Autodesk Inventor part; units mm, degrees
ref_plane "YZ Plane" through (0, 0, 0) normal (1, 0, 0) x (0, 1, 0)
ref_plane "XZ Plane" through (0, 0, 0) normal (0, 1, 0) x (-1, 0, 0)
ref_plane "XY Plane" through (0, 0, 0) normal (0, 0, 1) x (1, 0, 0)
sketch "Эскиз1" plane through (0, 0, 0) normal (0, 0, 1) x (1, 0, 0)
  line L0 (0, 0) -> (5.4, 0)
  line L1 (5.4, 0) -> (5.4, 4.4)
  line L2 (5.4, 4.4) -> (0, 4.4)
  line L3 (0, 4.4) -> (0, 0)
  dimension "d0" = 5.4
  dimension "d1" = 4.4
extrude "Выдавливание1" add sketch "Эскиз1" along normal blind 2
sketch "Эскиз2" plane through (0, 0, 2) normal (0, 0, 1) x (1, 0, 0)
  line L0 (0, 0) -> (5.4, 0)
  line L1 (5.4, 0) -> (5.4, 4.4)
  line L2 (5.4, 4.4) -> (0, 4.4)
  line L3 (0, 4.4) -> (0, 0)
  line L4 (0.3, 3.95) -> (5.1, 3.95)
  line L5 (5.1, 3.95) -> (5.1, 0.45)
  line L6 (5.1, 0.45) -> (0.3, 0.45)
  line L7 (0.3, 0.45) -> (0.3, 3.95)
  line L8 (-0.7, 4.95) -> (6.1, 4.95)
  line L9 (6.1, 4.95) -> (6.1, -0.55)
  line L10 (6.1, -0.55) -> (-0.7, -0.55)
  line L11 (-0.7, -0.55) -> (-0.7, 4.95)
  dimension "d4" = 4.8
  dimension "d5" = 3.5
  dimension "d6" = 5.4
  dimension "d7" = 4.4
  dimension "d8" = 0.3
  dimension "d9" = 0.45
  dimension "d12" = 1
  dimension "d13" = 1
  dimension "d14" = 1
  dimension "d15" = 1
extrude "Выдавливание3" add sketch "Эскиз2" along normal blind 1.5 contours L3 L2 L1 L0 | L8 L9 L10 L11
equation "\"d8\" = -0.5 * d4 + 0.5 * d6"
equation "\"d9\" = -0.5 * d5 + 0.5 * d7"
equation "\"d13\" = d12"
equation "\"d14\" = d12"
equation "\"d15\" = d12"
properties part number "button"
The listing builds one solid part. Answer for the finished solid, in the listing's coordinates (mm). A direction names the side the tool comes from. Coordinates: 2 decimals unless noted, no trailing zeros. Order: outer loops, then holes, each group sorted by start corner. A loop starts at its lowest first (then second) coordinate and runs counter-clockwise, first axis right, second up. Notation, with made-up numbers: M -33,40 L 15,40 A21 cw 15,78 Z; hole C 6,-34 d5. An arc over 180 degrees is marked long. Answer as a JSON object with one key per item and string values. Group by question number.
1. Determine the mould class of faces 4 (the flat face through (3, 0, 1)), 5 (the flat face through (3, 2, 2)), 6 (the flat face through (0.3, 2, 3)), 7 (the flat face through (0, 2, 1)) for opening direction Y: released by +Y, released by -Y, zero draft, split by the parting line, or undercut.
2. Section C-C on x = 4 is taken. Write down the section's boundary in (y, z), then the cut area to 3 significant figures.
3. Section A-A on z = 2.45 is taken. Write down the section's boundary in (x, y).
4. Straight lines are drawn through the part: line 1 (X direction, y = 3.25, z = 2.75); line 2 (Y direction, x = 4, z = 3.3); line 3 (Y direction, x = 0.75, z = 1.7). For each, find the intervals that lie inside material, in ascending order.
5. Section B-B on y = 0.1 is taken. Write down the section's boundary in (x, z), then the cut area to 3 significant figures.
6. Section D-D on z = 1.1 is taken. Write down the section's boundary in (x, y), then the cut area to 3 significant figures.
7. Flat-ended cylindrical pins translate along their axes: P1, Ø0.6, axis at y = 1.5, z = 1, coming from the -X side; P2, Ø1.8, axis at x = 1.5, y = 2, coming from the +Z side; P3, Ø1.6, axis at x = 2.5, z = 0.5, coming from the +Y side. Find the tip coordinate at first contact, or state that the pin passes through.
8. A tool of negligible diameter and unlimited length cuts with its end or side. For faces 1 (the flat face through (5.4, 2, 1)), 2 (the flat face through (3, 4.4, 1)), 3 (the flat face through (3, 3.95, 3)), from which of +Z, -Z, +X, -X, +Y, -Y can it reach the whole face along a straight path? Write none if from no direction.
Values follow:
{
 "1": {"face 4": "released by -Y", "face 5": "undercut", "face 6": "undercut", "face 7": "zero draft"},
 "2": {"outline": "M -0.55,2 L 0,2 L 0,0 L 4.4,0 L 4.4,2 L 4.95,2 L 4.95,3.5 L 3.95,3.5 L 3.95,2 L 0.45,2 L 0.45,3.5 L -0.55,3.5 Z", "area": "11.8 mm2"},
 "3": {"outline": "M -0.7,-0.55 L 6.1,-0.55 L 6.1,4.95 L -0.7,4.95 Z; hole M 0.3,0.45 L 5.1,0.45 L 5.1,3.95 L 0.3,3.95 Z"},
 "4": {"line 1": "-0.7 to 0.3, 5.1 to 6.1", "line 2": "-0.55 to 0.45, 3.95 to 4.95", "line 3": "0 to 4.4"},
 "5": {"outline": "M -0.7,2 L 0,2 L 0,0 L 5.4,0 L 5.4,2 L 6.1,2 L 6.1,3.5 L -0.7,3.5 Z", "area": "21.0 mm2"},
 "6": {"outline": "M 0,0 L 5.4,0 L 5.4,4.4 L 0,4.4 Z", "area": "23.8 mm2"},
 "7": {"P1": "x = 0", "P2": "z = 2", "P3": "y = 4.4"},
 "8": {"face 1": "-Z, +X, +Y, -Y", "face 2": "-Z, +X, -X, +Y", "face 3": "+Z"}
}
